from build123d import *

# Parameters (mm, degrees)
SKETCH1_R           = 1.5875
BOSS_EXTRUDE1_DEPTH = 9.525
SKETCH3_W           = 15
SKETCH3_H           = 3.175
SKETCH3_W_2         = 5
BOSS_EXTRUDE2_DEPTH = 12.7
FILLET1_R           = 6.35


with BuildPart() as part:
    # Sketch1 → Boss-Extrude1 (new body)
    with BuildSketch(Plane(origin=(0, 0, 0), x_dir=(0, 0, -1), z_dir=(1, 0, 0))):
        Polygon((0, 1.5875), (0, -1.5875), (-25.4, -1.5875), (-25.4, -4.7625), (-38.1, -4.7625), (-38.1, -1.5875), (-76.2, -1.5875), (-76.2, 1.5875), align=None)
        with Locations((-31.75, -1.5875)):
            Circle(SKETCH1_R, mode=Mode.SUBTRACT)
    extrude(amount=BOSS_EXTRUDE1_DEPTH)

    # Sketch3 → Boss-Extrude2 (add, symmetric)
    with BuildSketch(Plane(origin=(4.7625, 0, 0), x_dir=(0, 0, -1), z_dir=(1, 0, 0))):
        with Locations((-68.7, 0)):
            Rectangle(SKETCH3_W, SKETCH3_H)
        with Locations((-78.7, 0)):
            Rectangle(SKETCH3_W_2, SKETCH3_H)
    extrude(amount=BOSS_EXTRUDE2_DEPTH, both=True)

    # Fillet1
    fillet1_edges = [part.edges().sort_by_distance(p)[0] for p in [
        (0, 0, 61.2),
        (9.525, 0, 61.2),
    ]]
    fillet(fillet1_edges, radius=FILLET1_R)


solid = part.part
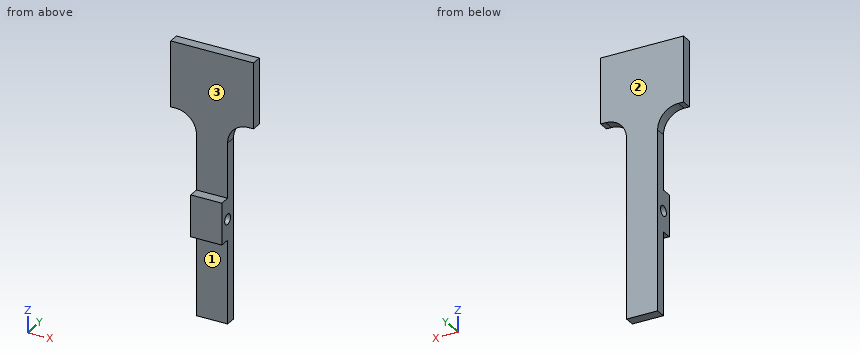
Model file for the job. Use its own axes, mm. Face numbers are marked on the shaded views. A direction names the side the tool comes from. Give positions to 0.01 mm unless a question says otherwise; leave off trailing zeros. Order: outer loops, then holes, each group sorted by start corner. A loop starts at its lowest first (then second) coordinate and runs counter-clockwise, first axis right, second up. Notation, with made-up numbers: (23.25, -8.5) - (36.25, -8.5) arc R15 cw to (36.25, 16.5) - close; hole circle Ø11 at (60, 41.25). An arc over 180 degrees is marked (long way). Return JSON: item names as keys, results as strings.
1) Cut at D-D, the plane x = -3. Give the cut face in (y, z), plus the area to 3 significant figures.
Geometry says:
{"outline": "(-1.59, 60.24) - (1.59, 60.24) - (1.59, 81.2) - (-1.59, 81.2) - close", "area": "66.5 mm²"}
2) Flat gauge pins, fed straight in: P1, Ø1.9, axis at y = -0.5, z = 15, coming from the -X side; P2, Ø1.3, axis at x = 16.5, y = 0, coming from the -Z side; P3, Ø5, axis at x = 3.5, z = 57.5, coming from the -Y side. Where does each tip first touch, or does it go through?
Geometry says:
{"P1": "x = 0", "P2": "z = 61.2", "P3": "y = -1.59"}
3) 3-axis set-ups, long thin cutter, end or side, ignore diameter. For the marked faces 1, 2 and 3: which of +Z, -Z, +X, -X, +Y, -Y reach the whole face in a straight line?
Geometry says:
{"face 1": "-Z, +X, -X, -Y", "face 2": "+Z, -Z, +X, -X, +Y", "face 3": "+Z, +X, -X, -Y"}
4) Cut at C-C, the plane z = 74. Give the cut face in (x, y), plus the area to 3 significant figures.
Geometry says:
{"outline": "(-7.94, -1.59) - (17.46, -1.59) - (17.46, 1.59) - (-7.94, 1.59) - close", "area": "80.6 mm²"}
5) Probe line 1 (Y direction, x = 4.25, z = 31.75) (1 decimal); line 2 (Z direction, x = 8.5, y = -1.75); line 3 (X direction, y = -3, z = 27) (3 decimals). List the from-to ranges inside material, lowest first. Write a range as from..to.
Geometry says:
{"line 1": "-4.8..-3.2, 0..1.6", "line 2": "25.4..30.17, 33.33..38.1", "line 3": "0..9.525"}
6) Cut at B-B, the plane z = 31.75. Give the cut face in (x, y) (1 decimal).
Geometry says:
{"outline": "(0, -4.8) - (9.5, -4.8) - (9.5, -3.2) - (0, -3.2) - close; (0, 0) - (9.5, 0) - (9.5, 1.6) - (0, 1.6) - close"}
